Source: CAD feature listing. Evaluate the final solid. Frame: model axes, mm. A direction names the side the tool comes from. Give positions to 0.01 mm unless a question says otherwise; leave off trailing zeros. Order: outer loops, then holes, each group sorted by start corner. A loop starts at its lowest first (then second) coordinate and runs counter-clockwise, first axis right, second up.
from build123d import *

# Parameters (mm, degrees)
SKETCH1_R           = 10
BOSS_EXTRUDE1_DEPTH = 5
SKETCH2_R           = 5.5
CUT_EXTRUDE1_DEPTH  = 2
SKETCH3_R           = 1.25
CUT_EXTRUDE2_DEPTH  = 2.5
FILLET1_R           = 1


with BuildPart() as part:
    # Sketch1 → Boss-Extrude1 (new body)
    with BuildSketch(Plane(origin=(0, 0, 0), x_dir=(1, 0, 0), z_dir=(0, 1, 0))):
        Circle(SKETCH1_R)
    extrude(amount=BOSS_EXTRUDE1_DEPTH)

    # Sketch2 → Cut-Extrude1 (cut)
    with BuildSketch(Plane(origin=(0, 5, 0), x_dir=(1, 0, 0), z_dir=(0, 1, 0))):
        Circle(SKETCH2_R)
    extrude(amount=-CUT_EXTRUDE1_DEPTH, mode=Mode.SUBTRACT)

    # Sketch3 → Cut-Extrude2 (cut)
    with BuildSketch(Plane.XZ):
        Circle(SKETCH3_R)
    extrude(amount=-CUT_EXTRUDE2_DEPTH, mode=Mode.SUBTRACT)

    # Fillet1
    fillet1_edges = [part.edges().sort_by_distance(p)[0] for p in [
        (-1.25, 2.5, 0),
    ]]
    fillet(fillet1_edges, radius=FILLET1_R)


solid = part.part
1) Section query A-A on x = -3. Output: boundary loops of the cut face in (y, z).
Checks:
outline: (0, -9.54) - (5, -9.54) - (5, -4.61) - (3, -4.61) - (3, 4.61) - (5, 4.61) - (5, 9.54) - (0, 9.54) - close
2) Section query C-C on y = 0.7. Output: boundary loops of the cut face in (x, z), and give its area (3 significant figures).
Checks:
outline: circle Ø20 at (0, 0); hole circle Ø2.5 at (0, 0)
area: 309 mm2
3) Ray query, L1, parallel to X at y = 3.7, z = -0.25; L2, parallel to Z at x = 0, y = 1.1. Return the intervals inside material, ascending.
Checks:
L1: x = -10 to -5.49, 5.49 to 10
L2: z = -10 to -1.25, 1.25 to 10
4) Section query D-D on y = 2.75. Output: boundary loops of the cut face in (x, z).
Checks:
outline: circle Ø20 at (0, 0)
5) Section query B-B on z = -5.25. Output: boundary loops of the cut face in (x, y).
Checks:
outline: (-8.51, 0) - (8.51, 0) - (8.51, 5) - (1.64, 5) - (1.64, 3) - (-1.64, 3) - (-1.64, 5) - (-8.51, 5) - close
6) First-contact query: pin 1 Ø3.5 at (x, z) = (-2, -0.5) entering from +Y; pin 2 Ø1.5 at (y, z) = (2.5, -3.5) entering from -X. Flat tips, straight axial feed; report the tip coordinate or a pass-through.
Checks:
pin 1: stops at y = 3
pin 2: stops at x = -9.61
7) Pull-direction query (Z, two-part tool) for faces 4 (the face through (0, 3, 0)), 5 (the face through (4, 5, 4)), 6 (the face through (-2.17, 2.46, 9.76)); classes: +Z half, -Z half, draft (parallel to the pull), parting line (faces both ways), or undercut.
Checks:
face 4: undercut
face 5: draft
face 6: parting line
8) Reachability of faces 1 (the face through (2, 0, 0)), 2 (the face through (-1.19, 4.01, 5.37)), 3 (the face through (-0.27, 0.74, -1.22)) from +Z, -Z, +X, -X, +Y, -Y: full face, straight path, thin tool, end or side. Return the list, or none.
Checks:
face 1: +Z, -Z, +X, -X, -Y
face 2: +Y
face 3: -Y
